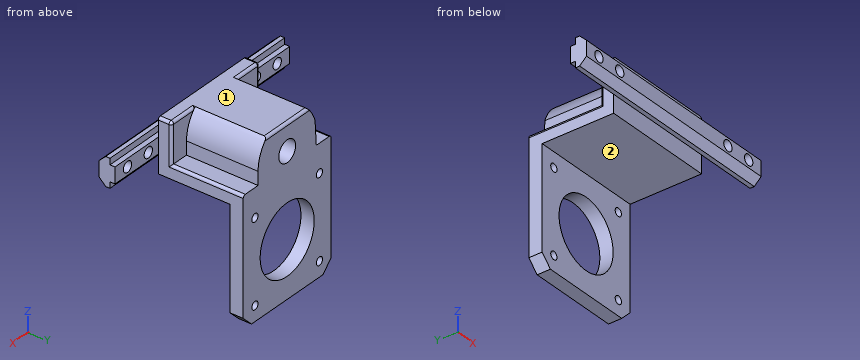
from build123d import *

# Parameters (mm, degrees)
BOSS_EXTRUDE1_DEPTH     = 42
SKETCH2_W               = 42.3
SKETCH2_H               = 20
BOSS_EXTRUDE2_DEPTH     = 32
SKETCH3_W               = 42.3
SKETCH3_H               = 42.3
BOSS_EXTRUDE3_DEPTH     = 5
SHELL2_START            = 11.1
SHELL2_OUTLINE_W        = 42.3
SHELL2_OUTLINE_H        = 15
SHELL2_DEPTH            = 27
CHAMFER2_SIZE           = 4
CUT_EXTRUDE1_DEPTH      = 75.799064165
CUT_EXTRUDE1_DEPTH_BACK = 75.799064165
SKETCH4_R               = 13
FILLET1_R               = 1
BOSS_EXTRUDE4_DEPTH     = 27
SKETCH18_R              = 4.05
CUT_EXTRUDE2_DEPTH      = 73.306915299
FILLET8_R               = 1
SKETCH19_R              = 1.5
CUT_EXTRUDE3_DEPTH      = 78.142076716
SKETCH20_R              = 2
CUT_EXTRUDE4_DEPTH      = 75.318840185


# Read off the part's stored shape, not the designer's step: Shell2
with BuildPart() as part:
    # Sketch1 → Boss-Extrude1 (new, symmetric)
    with BuildSketch(Plane(origin=(0, 0, 0), x_dir=(0, 0, -1), z_dir=(1, 0, 0))):
        Polygon((-3, 6.1), (3, 6.1), (3, 4.2), (5.3, 4.2), (5.3, 2.58), (2.8, 0), (-2.8, 0), (-5.3, 2.58), (-5.3, 4.2), (-3, 4.2), align=None)
    extrude(amount=BOSS_EXTRUDE1_DEPTH, both=True)

    # Sketch2 → Boss-Extrude2 (add)
    with BuildSketch(Plane(origin=(0, 6.1, 0), x_dir=(1, 0, 0), z_dir=(0, 1, 0))):
        Rectangle(SKETCH2_W, SKETCH2_H)
    extrude(amount=BOSS_EXTRUDE2_DEPTH)

    # Sketch3 → Boss-Extrude3 (add)
    with BuildSketch(Plane(origin=(0, 33.1, 0), x_dir=(1, 0, 0), z_dir=(0, 1, 0))):
        with Locations((0, 31.15)):
            Rectangle(SKETCH3_W, SKETCH3_H)
    extrude(amount=BOSS_EXTRUDE3_DEPTH)

    # Shell2 outline → Shell2 (cut)
    with BuildSketch(Plane(origin=(0, 0, 0), x_dir=(1, 0, 0), z_dir=(0, 1, 0)).offset(SHELL2_START)):
        with Locations((0, -2.5)):
            Rectangle(SHELL2_OUTLINE_W, SHELL2_OUTLINE_H)
    extrude(amount=SHELL2_DEPTH, mode=Mode.SUBTRACT)

    # Chamfer2
    chamfer2_edges = [part.edges().sort_by_distance(p)[0] for p in [
        (21.15, 35.6, -52.3),
        (-21.15, 35.6, -52.3),
    ]]
    chamfer(chamfer2_edges, length=CHAMFER2_SIZE)

    # Sketch4 → Cut-Extrude1 (cut, two sides: drawn at the far end of the back side and taken through both)
    with BuildSketch(Plane(origin=(0, 33.1, 0), x_dir=(1, 0, 0), z_dir=(0, 1, 0)).offset(-CUT_EXTRUDE1_DEPTH_BACK)):
        with Locations(Location((0, 31.15, 0), (0, 0, 270))):
            Circle(SKETCH4_R)
    extrude(amount=CUT_EXTRUDE1_DEPTH + CUT_EXTRUDE1_DEPTH_BACK, mode=Mode.SUBTRACT)

    # Fillet1
    fillet1_edges = [part.edges().sort_by_distance(p)[0] for p in [
        (-21.15, 8.6, 10),
        (21.15, 8.6, 10),
        (-21.15, 11.1, 2.5),
        (-21.15, 24.6, -5),
        (21.15, 11.1, 2.5),
        (21.15, 24.6, -5),
    ]]
    fillet(fillet1_edges, radius=FILLET1_R)

    # Sketch17 → Boss-Extrude4 (add)
    with BuildSketch(Plane(origin=(0, 11.1, 0), x_dir=(1, 0, 0), z_dir=(0, 1, 0))):
        with BuildLine():
            Line((14, 5), (-14, 5))
            Line((-14, 5), (-13.416407865, -4))
            ThreePointArc((-13.416407865, -4), (-11.98860738, -7.230027185), (-9.797958971, -10))
            Line((-9.797958971, -10), (9.797958971, -10))
            ThreePointArc((9.797958971, -10), (12.906808777, -5.423494003), (14, 0))
            Line((14, 0), (14, 5))
        make_face()
    extrude(amount=BOSS_EXTRUDE4_DEPTH)

    # Sketch18 → Cut-Extrude2 (cut, through all)
    with BuildSketch(Plane(origin=(0, 11.1, 0), x_dir=(1, 0, 0), z_dir=(0, 1, 0))):
        with Locations(Location((0, 0, 0), (0, 0, 270))):
            Circle(SKETCH18_R)
    extrude(amount=CUT_EXTRUDE2_DEPTH, mode=Mode.SUBTRACT)

    # Fillet8
    # the kernel refuses this fillet: 1 mm, written as the material it takes off along each edge
    with BuildSketch(Plane(origin=(-20.15, 10.1, 9), x_dir=(0, 1, 0), z_dir=(0, 0, 1))) as fillet8_piece_1_section:
        Polygon((0, 0), (FILLET8_R, 0), (FILLET8_R, FILLET8_R), (0, FILLET8_R), align=None)
    fillet8_piece_1 = extrude(amount=FILLET8_R, mode=Mode.PRIVATE)
    fillet8_piece_1 = fillet8_piece_1 - Plane(origin=(-20.15, 10.1, 9), x_dir=(0.7071067811865475, -0.7071067811865475, 0), z_dir=(0, 0, 1)) * Sphere(FILLET8_R, mode=Mode.PRIVATE)
    add(fillet8_piece_1, mode=Mode.SUBTRACT)
    with BuildSketch(Plane(origin=(20.15, 10.1, 9), x_dir=(0, 1, 0), z_dir=(0, 0, 1))) as fillet8_piece_2_section:
        Polygon((0, 0), (FILLET8_R, 0), (FILLET8_R, -FILLET8_R), (0, -FILLET8_R), align=None)
    fillet8_piece_2 = extrude(amount=FILLET8_R, mode=Mode.PRIVATE)
    fillet8_piece_2 = fillet8_piece_2 - Plane(origin=(20.15, 10.1, 9), x_dir=(-0.7071067811865475, -0.7071067811865475, 0), z_dir=(0, 0, 1)) * Sphere(FILLET8_R, mode=Mode.PRIVATE)
    add(fillet8_piece_2, mode=Mode.SUBTRACT)
    with BuildSketch(Plane(origin=(7.297958971, 11.1, 10), x_dir=(0, -1, 0), z_dir=(1, 0, 0))) as fillet8_piece_3_section:
        with BuildLine():
            CenterArc((FILLET8_R, FILLET8_R), FILLET8_R, 180, 90)
            Line((0, FILLET8_R), (0, 0))
            Line((0, 0), (FILLET8_R, 0))
        make_face()
    fillet8_piece_3 = extrude(amount=12.852041029, mode=Mode.PRIVATE)
    fillet8_piece_3 = fillet8_piece_3 - Plane(origin=(0, 10.87099501, 0), x_dir=(0.6998542122237654, 0, 0.7142857142857142), z_dir=(0, -1, 0)) * Cylinder(14, 30, mode=Mode.PRIVATE)
    add(fillet8_piece_3, mode=Mode.SUBTRACT)
    with BuildSketch(Plane(origin=(-12.297958971, 38.1, 10), x_dir=(0, 0, -1), z_dir=(1, 0, 0))) as fillet8_piece_4:
        with BuildLine():
            CenterArc((FILLET8_R, -FILLET8_R), FILLET8_R, 90, 90)
            Line((0, -FILLET8_R), (0, 0))
            Line((0, 0), (FILLET8_R, 0))
        make_face()
    extrude(amount=24.595917942, mode=Mode.SUBTRACT)
    with BuildSketch(Plane(origin=(-20.15, 11.1, 10), x_dir=(0, -1, 0), z_dir=(1, 0, 0))) as fillet8_piece_5_section:
        with BuildLine():
            CenterArc((FILLET8_R, FILLET8_R), FILLET8_R, 180, 90)
            Line((0, FILLET8_R), (0, 0))
            Line((0, 0), (FILLET8_R, 0))
        make_face()
    fillet8_piece_5 = extrude(amount=12.852041029, mode=Mode.PRIVATE)
    fillet8_piece_5 = fillet8_piece_5 - Plane(origin=(0, 10.870994427, 0), x_dir=(-0.9583148474999099, 0, 0.28571428571428575), z_dir=(0, -1, 0)) * Cylinder(14, 30, mode=Mode.PRIVATE)
    add(fillet8_piece_5, mode=Mode.SUBTRACT)

    # Sketch19 → Cut-Extrude3 (cut, through all)
    with BuildSketch(Plane(origin=(0, 38.1, 0), x_dir=(1, 0, 0), z_dir=(0, 1, 0))):
        with Locations(Location((-15.5, 46.65, 0), (0, 0, 270))):
            Circle(SKETCH19_R)
        with Locations(Location((15.5, 46.65, 0), (0, 0, 270))):
            Circle(SKETCH19_R)
        with Locations(Location((15.5, 15.65, 0), (0, 0, 270))):
            Circle(SKETCH19_R)
        with Locations(Location((-15.5, 15.65, 0), (0, 0, 270))):
            Circle(SKETCH19_R)
    extrude(amount=-CUT_EXTRUDE3_DEPTH, mode=Mode.SUBTRACT)

    # Sketch20 → Cut-Extrude4 (cut, through all)
    with BuildSketch(Plane(origin=(0, 6.1, 0), x_dir=(1, 0, 0), z_dir=(0, 1, 0))):
        with Locations(Location((36, 0, 0), (0, 0, 270))):
            Circle(SKETCH20_R)
        with Locations(Location((26, 0, 0), (0, 0, 270))):
            Circle(SKETCH20_R)
        with Locations(Location((-26, 0, 0), (0, 0, 270))):
            Circle(SKETCH20_R)
        with Locations(Location((-36, 0, 0), (0, 0, 270))):
            Circle(SKETCH20_R)
    extrude(amount=-CUT_EXTRUDE4_DEPTH, mode=Mode.SUBTRACT)


solid = part.part
For this review, take the finished solid that the model builds, in its own axes (mm). Face numbers are marked on the shaded views. A direction names the side the tool comes from. Give positions to 0.01 mm unless a question says otherwise; leave off trailing zeros. Loops run counter-clockwise (first coordinate to the right, second up) from the corner with the lowest first, then second, coordinate; pieces in that order, holes last. Notation, with made-up numbers: (-38.5, 26.5) -> (-0.5, 26.5) arc R4 cw to (-0.5, 33.5) -> close; hole circle Ø7 at (-6, -30.75). An arc over 180 degrees is marked (long way). One line per question, with ' | ' between items.
1) To check wall thickness, follow probe 1 along X at (y, z) = (4, 0); probe 2 along X at (y, z) = (34.2, -46.65); probe 3 along X at (y, z) = (35, -31). State the ranges of each line that lie inside material, in increasing order.
Resolved:
probe 1: x = -42 to -38, -34 to -28, -24 to 24, 28 to 34, 38 to 42 | probe 2: x = -21.15 to -17, -14 to 14, 17 to 21.15 | probe 3: x = -21.15 to -13, 13 to 21.15
2) We need section D-D (x = 0). Write out the cut boundary in (y, z), plus the area to 3 significant figures.
Resolved:
outline: (0, -2.8) -> (2.58, -5.3) -> (4.2, -5.3) -> (4.2, -3) -> (6.1, -3) -> (6.1, -10) -> (33.1, -10) -> (33.1, -18.15) -> (38.1, -18.15) -> (38.1, -4.05) -> (11.1, -4.05) -> (11.1, 4.05) -> (38.1, 4.05) -> (38.1, 9) arc R1 ccw to (37.1, 10) -> (6.1, 10) -> (6.1, 3) -> (4.2, 3) -> (4.2, 5.3) -> (2.58, 5.3) -> (0, 2.8) -> close; (33.1, -52.3) -> (38.1, -52.3) -> (38.1, -44.15) -> (33.1, -44.15) -> close | area: 552 mm2
3) Insertion check: pin 1 Ø4.5 at (x, z) = (-26, 0) entering from +Y; pin 2 Ø5 at (x, z) = (-15.5, -15.65) entering from -Y; pin 3 Ø0.9 at (x, y) = (3, 5.5) entering from -Z; pin 4 Ø2.5 at (x, z) = (-36, 0) entering from -Y. Each pin has a flat end and moves straight along its axis. Give the tip position at first contact, or say it passes through.
Resolved:
pin 1: stops at y = 6.1 | pin 2: stops at y = 33.1 | pin 3: stops at z = -3 | pin 4: passes through
4) We need section A-A (x = -15.5). Write out the cut boundary in (y, z).
Resolved:
outline: (0, -2.8) -> (2.58, -5.3) -> (4.2, -5.3) -> (4.2, -3) -> (6.1, -3) -> (6.1, -10) -> (33.1, -10) -> (33.1, -14.15) -> (38.1, -14.15) -> (38.1, -5) -> (11.1, -5) -> (11.1, 9) arc R1 ccw to (10.1, 10) -> (6.1, 10) -> (6.1, 3) -> (4.2, 3) -> (4.2, 5.3) -> (2.58, 5.3) -> (0, 2.8) -> close; (33.1, -52.3) -> (38.1, -52.3) -> (38.1, -48.15) -> (33.1, -48.15) -> close; (33.1, -45.15) -> (38.1, -45.15) -> (38.1, -17.15) -> (33.1, -17.15) -> close
5) For the marked faces 1 and 2, list the 3-axis set-ups (+Z, -Z, +X, -X, +Y, -Y) from which the entire face can be reached by the end or side of a thin tool; tool diameter is ignored.
Resolved:
face 1: +Z, +X, -X, +Y, -Y | face 2: -Z, +X, -X, -Y
6) We need section C-C (y = 28). Write out the cut boundary in (x, z).
Resolved:
outline: (-21.15, -10) -> (21.15, -10) -> (21.15, -6) arc R1 ccw to (20.15, -5) -> (14, -5) -> (14, 0) arc R14 ccw to (9.8, 10) -> (-9.8, 10) arc R14 ccw to (-13.42, 4) -> (-14, -5) -> (-20.15, -5) arc R1 ccw to (-21.15, -6) -> close; hole circle Ø8.1 at (0, 0)
7) We need section B-B (z = -31.15). Write out the cut boundary in (x, y), plus the area to 3 significant figures.
Resolved:
outline: (-21.15, 33.1) -> (-13, 33.1) -> (-13, 38.1) -> (-21.15, 38.1) -> close; (13, 33.1) -> (21.15, 33.1) -> (21.15, 38.1) -> (13, 38.1) -> close | area: 81.5 mm2
